Read the model definition and answer for the solid it produces. Units are mm, in the model's axes. A direction names the side the tool comes from. Coordinates: 2 decimals unless noted, no trailing zeros. Write each loop counter-clockwise with the first axis right and the second up, starting at its lowest first coordinate (ties: lowest second). Pieces come first, ordered by that corner, then holes.
(1) The mould has two halves that part along X. Classify faces 5 (the flat face through (374.396, 65, -354)), 6 (the flat face through (256.7, 43, -354)), 7 (the flat face through (262, 69.999, -354)), 8 (the flat face through (269.875, 66, -354)): +X half, -X half, draft (parallel to the pull), parting line (faces both ways), or undercut.
(2) Given pin 1 (1.5 mm diameter, centred on x = 261.5, z = -355, fed in from +Y); pin 2 (1.5 mm diameter, centred on x = 298, z = -355, fed in from -Y); pin 3 (1.5 mm diameter, centred on x = 378, z = -354.5, fed in from +Y), each flat-ended and moving along its own axis, determine where each tip first touches the part or whether it passes through.
(3) Which of the six approach directions +Z, -Z, +X, -X, +Y, -Y give full straight-line access (tool end or side, diameter ignored) to faces 1 (the flat face through (373, 61.521, -354)), 2 (the flat face through (365, 16.439, -354)), 3 (the flat face through (344.221, 31, -354)), 4 (the flat face through (379, 69.125, -354))?
(4) Section C-C on x = 362 is taken. Write down the section's boundary in (y, z), then the cut area to 3 significant figures.
(5) Section A-A on y = 32 is taken. Write down the section's boundary in (x, z) (3 decimals), then the cut area to 3 significant figures.
(6) Find the intervals of material crossed by probe 1 along X at (y, z) = (33, -353.35) (3 decimals); probe 2 along X at (y, z) = (64.5, -354.65) (3 decimals); probe 3 along X at (y, z) = (63, -354.05) (3 decimals), in increasing order.
(7) Section B-B on z = -354 is taken. Write down the section's boundary in (x, y) (3 decimals), then the cut area to 3 significant figures.
from build123d import *

# Parameters (mm, degrees)
BOSS_EXTRUDE1_DEPTH = 3


with BuildPart() as part:
    # Sketch2 → Boss-Extrude1 (new body)
    with BuildSketch(Plane.XY.offset(-353)):
        Polygon((371.221, 61.521478107), (374.396, 61.521478107), (374.396, 69.124950745), (384.396, 69.124950745), (384.396, 16.438825445), (344.221, 16.438825445), (344.221, 46.438825445), (341.221, 46.438825445), (341.221, 16.438825445), (299.875, 16.438825445), (299.875, 46.438825445), (296.875, 46.438825445), (296.875, 16.438825445), (256.7, 16.438825445), (256.7, 69.999273471), (266.7, 69.999273471), (266.7, 62.349211745), (269.875, 62.349211745), (269.875, 69.999275879), (318.872542602, 70.779885056), (319.031094476, 63.13005689), (322.205416715, 63.195722676), (322.046864787, 70.845553451), (371.221, 69.124947668), align=None)
    extrude(amount=-BOSS_EXTRUDE1_DEPTH)


solid = part.part
Response:
1. face 5: undercut
1. face 6: -X half
1. face 7: draft
1. face 8: undercut
2. pin 1: stops at y = 70
2. pin 2: stops at y = 46.44
2. pin 3: stops at y = 69.12
3. face 1: +Z, -Z, +Y
3. face 2: +Z, -Z, +X, -X, -Y
3. face 3: +Z, -Z, -Y
3. face 4: +Z, -Z, +X, +Y
4. outline: (16.44, -356) - (69.45, -356) - (69.45, -353) - (16.44, -353) - close
4. area: 159 mm2
5. outline: (256.7, -356) - (296.875, -356) - (296.875, -353) - (256.7, -353) - close; (299.875, -356) - (341.221, -356) - (341.221, -353) - (299.875, -353) - close; (344.221, -356) - (384.396, -356) - (384.396, -353) - (344.221, -353) - close
5. area: 365 mm2
6. probe 1: x = 256.7 to 296.875, 299.875 to 341.221, 344.221 to 384.396
6. probe 2: x = 256.7 to 266.7, 269.875 to 319.003, 322.178 to 371.221, 374.396 to 384.396
6. probe 3: x = 256.7 to 266.7, 269.875 to 371.221, 374.396 to 384.396
7. outline: (256.7, 16.439) - (296.875, 16.439) - (296.875, 46.439) - (299.875, 46.439) - (299.875, 16.439) - (341.221, 16.439) - (341.221, 46.439) - (344.221, 46.439) - (344.221, 16.439) - (384.396, 16.439) - (384.396, 69.125) - (374.396, 69.125) - (374.396, 61.521) - (371.221, 61.521) - (371.221, 69.125) - (322.047, 70.846) - (322.205, 63.196) - (319.031, 63.13) - (318.873, 70.78) - (269.875, 69.999) - (269.875, 62.349) - (266.7, 62.349) - (266.7, 69.999) - (256.7, 69.999) - close
7. area: 6,600 mm2
